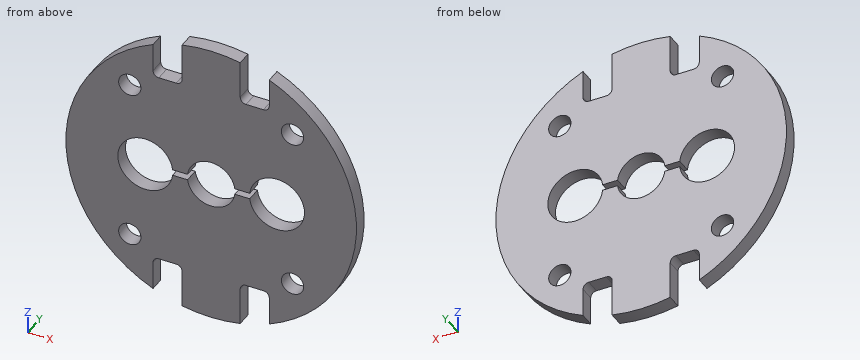
```python
from build123d import *

# Parameters (mm, degrees)
BOSS_EXTRUDE1_DEPTH       = 0.8
CUT_EXTRUDE1_DEPTH        = 2.6
F_2_CLEARANCE_HOLE1_D     = 2.4384
F_2_CLEARANCE_HOLE1_DEPTH = 1.6


with BuildPart() as part:
    # Sketch1 → Boss-Extrude1 (new body, symmetric)
    with BuildSketch(Plane(origin=(0, 0, 0), x_dir=(1, 0, 0), z_dir=(0, 1, 0))):
        with BuildLine():
            Line((-6.35, 14.549677831), (-6.35, 11.43))
            ThreePointArc((-6.35, 11.43), (-6.164012806, 10.980987194), (-5.715, 10.795))
            Line((-5.715, 10.795), (-3.81, 10.795))
            ThreePointArc((-3.81, 10.795), (-3.360987194, 10.980987194), (-3.175, 11.43))
            Line((-3.175, 11.43), (-3.175, 15.554259867))
            ThreePointArc((-3.175, 15.554259867), (0, 15.875), (3.175, 15.554259867))
            Line((3.175, 15.554259867), (3.175, 11.43))
            ThreePointArc((3.175, 11.43), (3.360987194, 10.980987194), (3.81, 10.795))
            Line((3.81, 10.795), (5.715, 10.795))
            ThreePointArc((5.715, 10.795), (6.164012806, 10.980987194), (6.35, 11.43))
            Line((6.35, 11.43), (6.35, 14.549677831))
            ThreePointArc((6.35, 14.549677831), (15.875, 0), (6.35, -14.549677831))
            Line((6.35, -14.549677831), (6.35, -11.43))
            ThreePointArc((6.35, -11.43), (6.164012806, -10.980987194), (5.715, -10.795))
            Line((5.715, -10.795), (3.81, -10.795))
            ThreePointArc((3.81, -10.795), (3.360987194, -10.980987194), (3.175, -11.43))
            Line((3.175, -11.43), (3.175, -15.554259867))
            ThreePointArc((3.175, -15.554259867), (0, -15.875), (-3.175, -15.554259867))
            Line((-3.175, -15.554259867), (-3.175, -11.43))
            ThreePointArc((-3.175, -11.43), (-3.360987194, -10.980987194), (-3.81, -10.795))
            Line((-3.81, -10.795), (-5.715, -10.795))
            ThreePointArc((-5.715, -10.795), (-6.164012806, -10.980987194), (-6.35, -11.43))
            Line((-6.35, -11.43), (-6.35, -14.549677831))
            ThreePointArc((-6.35, -14.549677831), (-15.875, 0), (-6.35, 14.549677831))
        make_face()
    extrude(amount=BOSS_EXTRUDE1_DEPTH, both=True)

    # Sketch2 → Cut-Extrude1 (cut, through all)
    with BuildSketch(Plane(origin=(0, 0.8, 0), x_dir=(1, 0, 0), z_dir=(0, 1, 0))):
        with BuildLine():
            Line((-4.217656123, 0.325), (-2.579607528, 0.325))
            ThreePointArc((-2.579607528, 0.325), (0, 2.6), (2.579607528, 0.325))
            Line((2.579607528, 0.325), (4.217656123, 0.325))
            ThreePointArc((4.217656123, 0.325), (10.2, 0), (4.217656123, -0.325))
            Line((4.217656123, -0.325), (2.579607528, -0.325))
            ThreePointArc((2.579607528, -0.325), (0, -2.6), (-2.579607528, -0.325))
            Line((-2.579607528, -0.325), (-4.217656123, -0.325))
            ThreePointArc((-4.217656123, -0.325), (-10.2, 0), (-4.217656123, 0.325))
        make_face()
    extrude(amount=-CUT_EXTRUDE1_DEPTH, mode=Mode.SUBTRACT)

    # #2 Clearance Hole1
    with Locations(Plane(origin=(0, 0.8, 0), x_dir=(1, 0, 0), z_dir=(0, 1, 0))):
        with Locations((-8.89, 8.89), (8.89, 8.89), (-8.89, -8.89), (8.89, -8.89)):
            Hole(F_2_CLEARANCE_HOLE1_D / 2, depth=F_2_CLEARANCE_HOLE1_DEPTH)


solid = part.part
```
Geometry check sheet. Reference: the model listing, model coordinates, mm. Give positions to 0.01 mm unless a question says otherwise; leave off trailing zeros. Order: outer loops, then holes, each group sorted by start corner. A loop starts at its lowest first (then second) coordinate and runs counter-clockwise, first axis right, second up.
1. Section check A-A, the plane z = 8.89. Enter the section's corners in (x, y), and give its area (3 significant figures).
2. Section check B-B, the plane x = -5. Enter the section's corners in (y, z) (3 decimals), and give its area (3 significant figures).
3. Section check D-D, the plane y = -0.5. Give the number of separate pieces and of enclosed holes in the cut face, and give its area (3 significant figures).
4. Gauge pin test, flat ends, axial feed: pin 1 Ø5.5 at (x, z) = (7.2, 0) entering from -Y; pin 2 Ø0.8 at (y, z) = (0, -13) entering from +X; pin 3 Ø0.8 at (y, z) = (-0.5, 13.5) entering from +X. Record the tip position at first contact, or that the pin passes through.
5. Section check C-C, the plane x = -8.89. Enter the section's corners in (y, z), and give its area (3 significant figures).
6. Thickness scan on L1, parallel to Z at x = 8.89, y = 0.3; L2, parallel to X at y = 0.2, z = -8.89; L3, parallel to X at y = 0.5, z = -8. Record the ranges inside material, lowest first.
Values follow:
1. outline: (-13.15, -0.8) - (-10.11, -0.8) - (-10.11, 0.8) - (-13.15, 0.8) - close; (-7.67, -0.8) - (7.67, -0.8) - (7.67, 0.8) - (-7.67, 0.8) - close; (10.11, -0.8) - (13.15, -0.8) - (13.15, 0.8) - (10.11, 0.8) - close
1. area: 34.3 mm2
2. outline: (-0.8, -10.795) - (0.8, -10.795) - (0.8, -2.04) - (-0.8, -2.04) - close; (-0.8, 2.04) - (0.8, 2.04) - (0.8, 10.795) - (-0.8, 10.795) - close
2. area: 28.0 mm2
3. separate pieces: 1
3. enclosed holes: 5
3. area: 639 mm2
4. pin 1: passes through
4. pin 2: stops at x = 9.66
4. pin 3: stops at x = 8.97
5. outline: (-0.8, -13.15) - (0.8, -13.15) - (0.8, -10.11) - (-0.8, -10.11) - close; (-0.8, -7.67) - (0.8, -7.67) - (0.8, -2.48) - (-0.8, -2.48) - close; (-0.8, 2.48) - (0.8, 2.48) - (0.8, 7.67) - (-0.8, 7.67) - close; (-0.8, 10.11) - (0.8, 10.11) - (0.8, 13.15) - (-0.8, 13.15) - close
5. area: 26.4 mm2
6. L1: z = -13.15 to -10.11, -7.67 to -2.48, 2.48 to 7.67, 10.11 to 13.15
6. L2: x = -13.15 to -10.11, -7.67 to 7.67, 10.11 to 13.15
6. L3: x = -13.71 to -9.72, -8.06 to 8.06, 9.72 to 13.71
